from build123d import *

# Parameters (mm, degrees)
F1_DEPTH = 38.1
F3_DEPTH = 44.45
F4_W     = 1.4423634857
F4_H     = 16.5442936122
F5_DEPTH = 12.7
F4_W_2   = 1.6968995333
F6_DEPTH = 12.7


with BuildPart() as f1:
    # F0 (on Front) → F1 (new body)
    with BuildSketch(Plane.XZ):
        with BuildLine():
            Line((-25.10883745, 38.448043143), (-24.820253253, 0))
            ThreePointArc((-24.820253253, 0), (-0.1008948311, -24.534515601), (24.6184635907, 0))
            Line((24.6184635907, 0), (24.6184635907, 38.8212874506))
            Line((24.6184635907, 38.8212874506), (-25.10883745, 38.448043143))
        make_face()
    extrude(amount=F1_DEPTH)

    # F2 (on face) → F3 (cut)
    with BuildSketch(Plane(origin=(-0.2899824262, 0, 38.6343290697), x_dir=(0.9999718325, 0, 0.0075056113), z_dir=(-0.0075056113, 0, 0.9999718325))):
        with BuildLine():
            Line((-16.7144715449, -35.4128060373), (16.2133492063, -35.4128060373))
            ThreePointArc((16.2133492063, -35.4128060373), (21.4057154297, -19.1007387378), (16.2469655347, -2.7780089998))
            Line((16.2469655347, -2.7780089998), (-16.7454987534, -2.7780089998))
            ThreePointArc((-16.7454987534, -2.7780089998), (-21.5733199015, -19.1000122708), (-16.7144715449, -35.4128060373))
        make_face()
    extrude(amount=-F3_DEPTH, mode=Mode.SUBTRACT)

    # F4 (on face) → F5 (cut)
    with BuildSketch(Plane(origin=(-0.2899824262, 0, 38.6343290697), x_dir=(0.9999718325, 0, 0.0075056113), z_dir=(-0.0075056113, 0, 0.9999718325))):
        with Locations((-23.0341581628, -17.9296452552)):
            Rectangle(F4_W, F4_H)
    extrude(amount=-F5_DEPTH, mode=Mode.SUBTRACT)

    # F4 (on face) → F6 (cut)
    with BuildSketch(Plane(origin=(-0.2899824262, 0, 38.6343290697), x_dir=(0.9999718325, 0, 0.0075056113), z_dir=(-0.0075056113, 0, 0.9999718325))):
        with Locations((-23.0341581628, -17.9296452552)):
            Rectangle(F4_W, F4_H)
        with Locations((22.6548295468, -17.9296452552)):
            Rectangle(F4_W_2, F4_H)
    extrude(amount=-F6_DEPTH, mode=Mode.SUBTRACT)


solid = f1.part
The listing builds one solid part. Answer for the finished solid, in the listing's coordinates (mm). A direction names the side the tool comes from. Round coordinates to 2 decimals unless told otherwise and drop trailing zeros. Write each loop counter-clockwise with the first axis right and the second up, starting at its lowest first coordinate (ties: lowest second). Pieces come first, ordered by that corner, then holes. Notation, with made-up numbers: (74, -29.75) - (105, -29.75) arc R32 cw to (105, -3.75) - close; hole circle Ø7 at (72, 42). An arc over 180 degrees is marked (long way). Use one line per item in the form item = value. Start each with the question number.
Item 1: Determine the mould class of faces 3 (the cylindrical face through (21.28, -19.34, 16.88)), 4 (the flat face through (24.618, -19, 19)), 5 (the flat face through (-1, -38.1, 8)), 6 (the flat face through (22, -9.657, 33)) for opening direction Y: +Y half, -Y half, draft (parallel to the pull), parting line (faces both ways), or undercut.
Item 2: A cutting plane is placed at A-A (x = 3). Write down the section's boundary in (y, z).
Item 3: A cutting plane is placed at D-D (x = -13). Write down the section's boundary in (y, z).
Item 4: A cutting plane is placed at C-C (z = 33.5). Give the number of separate pieces and of enclosed holes in the cut face, plus the area to 3 significant figures.
Item 5: A tool of negligible diameter and unlimited length cuts with its end or side. For faces 1 (the flat face through (-1, -35.413, 17)), 2 (the cylindrical face through (-0.64, -18.78, -24.53)), from which of +Z, -Z, +X, -X, +Y, -Y can it reach the whole face along a straight path? Write none if from no direction.
Item 6: Find the intervals of material crossed by line 1 (Y direction, x = 16, z = 23); line 2 (X direction, y = -16, z = 33); line 3 (X direction, y = -20, z = 16.5), in increasing order. Write a range as [from, to].
Item 7: Flat-ended cylindrical pins translate along their axes: pin 1 Ø2 at (x, z) = (22, 35) entering from +Y; pin 2 Ø1 at (x, y) = (16, -22.5) entering from -Z; pin 3 Ø2 at (y, z) = (-13, -12) entering from -X; pin 4 Ø1.5 at (x, y) = (-17.5, -11.5) entering from +Z. Find the tip coordinate at first contact, or state that the pin passes through.
The answers:
q1.face_3 = undercut
q1.face_4 = draft
q1.face_5 = -Y half
q1.face_6 = undercut
q2.outline = (-38.1, -24.34) - (0, -24.34) - (0, 38.66) - (-2.78, 38.66) - (-2.78, -5.79) - (-35.41, -5.79) - (-35.41, 38.66) - (-38.1, 38.66) - close
q3.outline = (-38.1, -20.9) - (0, -20.9) - (0, 38.54) - (-2.78, 38.54) - (-2.78, -5.91) - (-35.41, -5.91) - (-35.41, 38.54) - (-38.1, 38.54) - close
q4.separate_pieces = 1
q4.enclosed_holes = 3
q4.area = 544 mm^2
q5.face_1 = +Z
q5.face_2 = -Z, +Y, -Y
q6.line_1 = [-38.1, -35.41], [-2.78, 0]
q6.line_2 = [-25.07, -24], [-22.56, -21.66], [20.99, 21.56], [23.26, 24.62]
q6.line_3 = [-24.94, -21.68], [21.27, 24.62]
q7.pin_1 = 0
q7.pin_2 = -18.99
q7.pin_3 = -22.15
q7.pin_4 = -5.94
